The figure shows three views and two pictorial views of one solid part (mm, origin at its lowest corner). Answer the questions. A direction names the side the tool comes from. Coordinates: 2 decimals unless noted, no trailing zeros. Write each loop counter-clockwise with the first axis right and the second up, starting at its lowest first coordinate (ties: lowest second). Pieces come first, ordered by that corner, then holes.
Item 1: Section B-B (y = 12.5) is taken. State how many separate pieces and enclosed holes the cut face has, then the cut area to 3 significant figures.
Item 2: Section D-D (y = 31.67) is taken. Give the vertices of the cut face in (x, z).
Item 3: Section C-C (z = 40.4) is taken. Give the vertices of the cut face in (x, y), then the cut area to 3 significant figures.
Item 4: Section A-A (x = 25.4) is taken. Give the vertices of the cut face in (y, z), then the cut area to 3 significant figures.
Item 5: Straight lines are drawn through the part: probe 1 along Y at (x, z) = (2, 40); probe 2 along Y at (x, z) = (48.6, 10.4); probe 3 along Y at (x, z) = (25, 50). For each, find the intervals that lie inside material, in ascending order.
Item 6: A tool of negligible diameter and unlimited length cuts with its end or side. For the marked faces 1 and 2, from which of +Z, -Z, +X, -X, +Y, -Y can it reach the whole face along a straight path? Write none if from no direction.
Item 7: Determine the mould class of the marked faces 3, 4, 5 and 6 for opening direction X: released by +X, released by -X, zero draft, split by the parting line, or undercut.
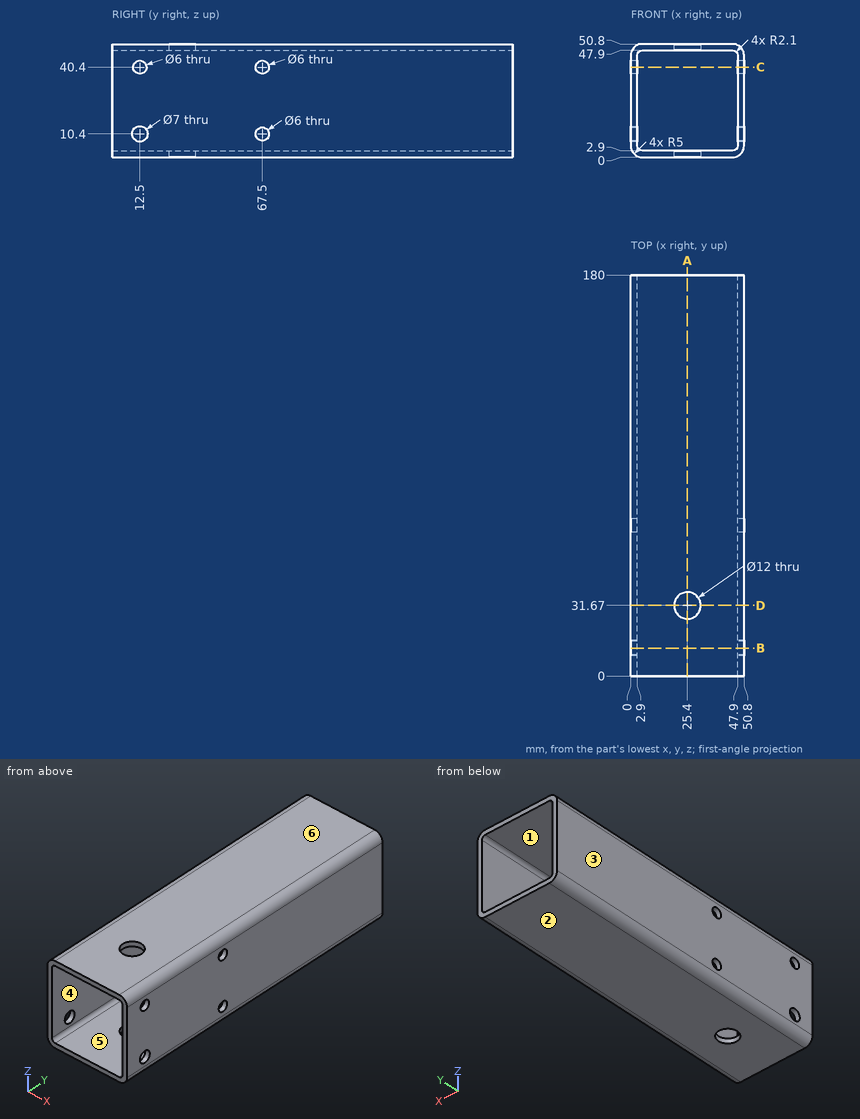
Established:
1. separate pieces: 4
1. enclosed holes: 0
1. area: 463 mm2
2. outline: (0, 5) arc R5 ccw to (5, 0) - (19.4, 0) - (19.4, 2.9) - (5, 2.9) arc R2.1 cw to (2.9, 5) - (2.9, 45.8) arc R2.1 cw to (5, 47.9) - (19.4, 47.9) - (19.4, 50.8) - (5, 50.8) arc R5 ccw to (0, 45.8) - close; (31.4, 0) - (45.8, 0) arc R5 ccw to (50.8, 5) - (50.8, 45.8) arc R5 ccw to (45.8, 50.8) - (31.4, 50.8) - (31.4, 47.9) - (45.8, 47.9) arc R2.1 cw to (47.9, 45.8) - (47.9, 5) arc R2.1 cw to (45.8, 2.9) - (31.4, 2.9) - close
3. outline: (0, 0) - (2.9, 0) - (2.9, 9.5) - (0, 9.5) - close; (0, 15.5) - (2.9, 15.5) - (2.9, 64.5) - (0, 64.5) - close; (0, 70.5) - (2.9, 70.5) - (2.9, 180) - (0, 180) - close; (47.9, 0) - (50.8, 0) - (50.8, 9.5) - (47.9, 9.5) - close; (47.9, 15.5) - (50.8, 15.5) - (50.8, 64.5) - (47.9, 64.5) - close; (47.9, 70.5) - (50.8, 70.5) - (50.8, 180) - (47.9, 180) - close
3. area: 974 mm2
4. outline: (0, 0) - (25.67, 0) - (25.67, 2.9) - (0, 2.9) - close; (0, 47.9) - (25.67, 47.9) - (25.67, 50.8) - (0, 50.8) - close; (37.67, 0) - (180, 0) - (180, 2.9) - (37.67, 2.9) - close; (37.67, 47.9) - (180, 47.9) - (180, 50.8) - (37.67, 50.8) - close
4. area: 974 mm2
5. probe 1: y = 0 to 9.53, 15.47 to 64.53, 70.47 to 180
5. probe 2: y = 0 to 9, 16 to 64.5, 70.5 to 180
5. probe 3: y = 0 to 25.68, 37.66 to 180
6. face 1: +Y, -Y
6. face 2: -Z, +X, -X, +Y, -Y
7. face 3: released by -X
7. face 4: undercut
7. face 5: undercut
7. face 6: zero draft
